Design review of the part built by this model. Coordinates are the model's own, in mm. Face numbers are marked on the shaded views. Coordinates: 2 decimals unless noted, no trailing zeros. Write each loop counter-clockwise with the first axis right and the second up, starting at its lowest first coordinate (ties: lowest second). Pieces come first, ordered by that corner, then holes.
Q1. Take a section at D-D, the plane z = 7. Write out the cut boundary in (x, y).
Q2. For pin 1 Ø4 at (x, z) = (0, 6.5) entering from -Y; pin 2 Ø3 at (x, z) = (0, 0) entering from -Y; pin 3 Ø1.6 at (x, z) = (-1, 10.5) entering from +Y, all flat-tipped, find the tip position at first contact; note any pin that passes through.
Q3. For L1, parallel to Z at x = 0, y = 4.65; L2, parallel to Y at x = -2, z = 9; L3, parallel to Z at x = -1, y = 2.95, list the stretches that pass through material, from the lowest coordinate up.
Q4. The part is to be moulded in two halves that separate along X. For the marked faces 1, 2 and 3, say which applies: released by +X, released by -X, zero draft, split by the parting line, or undercut.
Q5. Take a section at A-A, the plane x = 0. Write out the cut boundary in (y, z), plus the area to 3 significant figures.
Q6. Take a section at B-B, the plane z = 0. Write out the cut boundary in (x, y).
Q7. Take a section at C-C, the plane y = 0.9. Write out the cut boundary in (x, z), plus the area to 3 significant figures.
Autodesk Inventor part; units mm, degrees
ref_plane "Work Plane1" through (0, 4.4, 0) normal (0, 1, 0) x (1, 0, 0)
ref_plane "YZ Plane" through (0, 0, 0) normal (1, 0, 0) x (0, 1, 0)
ref_plane "XZ Plane" through (0, 0, 0) normal (0, 1, 0) x (-1, 0, 0)
sketch "Sketch1" plane through (0, 0, 0) normal (0, 1, 0) x (-1, 0, 0)
  circle A0 centre (0, 0) radius 3.35
  dimension "d0" = 6.7
extrude "Extrusion1" add sketch "Sketch1" along normal blind 4.8
ref_plane "Work Plane1" through (0, 4.4, 0) normal (0, 1, 0) x (1, 0, 0)
sketch "Sketch2" plane through (0, 4.4, 0) normal (0, 1, 0) x (1, 0, 0)
  circle A0 centre (0, 0) radius 3.35
  line L0 (-2.6, 2.1125) -> (-2, 13.453)
  circle A1 centre (0, 0) radius 3.35
  line L1 (2.6, 2.1125) -> (2, 13.453)
  arc A2 (2, 13.453) -> (-2, 13.453) centre (0, 13.3472) ccw
  line L2 (-2, 13.453) -> (2, 13.453) construction
  line L3 (2.6, 2.1125) -> (-2.6, 2.1125) construction
  line L4 (0, 0) -> (-1.2831, 0)
  line L5 (-2.6, -2.1125) -> (-2, -13.453)
  line L6 (2.6, -2.1125) -> (2, -13.453)
  arc A3 (-2, -13.453) -> (2, -13.453) centre (0, -13.3472) ccw
  line L7 (-2, -13.453) -> (2, -13.453) construction
  line L8 (2.6, -2.1125) -> (-2.6, -2.1125) construction
  dimension "d4" = 5.2
  dimension "d5" = 12
  dimension "d6" = 4
extrude "Extrusion2" add sketch "Sketch2" against normal blind 2.2 contours A0 L0 A2 L1 | L6 A3 L5 A0
sketch "Sketch3" plane through (0, 4.8, 0) normal (0, 1, 0) x (1, 0, 0)
  circle A0 centre (0, 0) radius 1.25
  circle A1 centre (0, 0) radius 2.3
  dimension "d9" = 2.5
  dimension "d10" = 4.6
extrude "Extrusion3" cut sketch "Sketch3" against normal through all contours A0
extrude "Extrusion4" cut sketch "Sketch3" against normal blind 1
sketch "Sketch4" plane through (0, 0, 0) normal (0, -1, 0) x (1, 0, 0)
  circle A0 centre (0, 0) radius 2.35
  dimension "d15" = 4.7
extrude "Extrusion5" cut sketch "Sketch4" against normal blind 2.9
properties part number "attachmnet" material "Nylon 6/6"
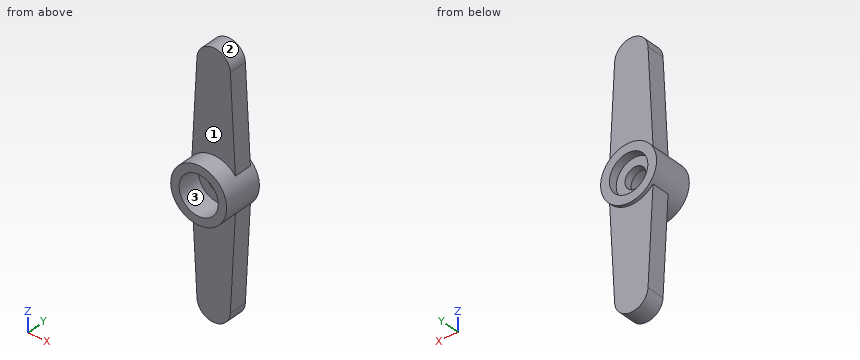
Responses:
1. outline: (-2.34, 2.2) - (2.34, 2.2) - (2.34, 4.4) - (-2.34, 4.4) - close
2. pin 1: stops at y = 2.2
2. pin 2: stops at y = 2.9
2. pin 3: stops at y = 4.4
3. L1: z = -3.35 to -2.3, 2.3 to 3.35
3. L2: y = 2.2 to 4.4
3. L3: z = -15.08 to -0.75, 0.75 to 15.08
4. face 1: zero draft
4. face 2: split by the parting line
4. face 3: undercut
5. outline: (0, -3.35) - (2.2, -3.35) - (2.2, -15.35) - (4.4, -15.35) - (4.4, -3.35) - (4.8, -3.35) - (4.8, -2.3) - (3.8, -2.3) - (3.8, -1.25) - (2.9, -1.25) - (2.9, -2.35) - (0, -2.35) - close; (0, 2.35) - (2.9, 2.35) - (2.9, 1.25) - (3.8, 1.25) - (3.8, 2.3) - (4.8, 2.3) - (4.8, 3.35) - (4.4, 3.35) - (4.4, 15.35) - (2.2, 15.35) - (2.2, 3.35) - (0, 3.35) - close
5. area: 64.5 mm2
6. outline: (-3.35, 0) - (-2.35, 0) - (-2.35, 2.9) - (-1.25, 2.9) - (-1.25, 3.8) - (-2.3, 3.8) - (-2.3, 4.8) - (-3.35, 4.8) - close; (1.25, 2.9) - (2.35, 2.9) - (2.35, 0) - (3.35, 0) - (3.35, 4.8) - (2.3, 4.8) - (2.3, 3.8) - (1.25, 3.8) - close
7. outline: circle Ø6.7 at (0, 0); hole circle Ø4.7 at (0, 0)
7. area: 17.9 mm2
